Autodesk Inventor part; units mm, degrees
ref_plane "YZ Plane" through (0, 0, 0) normal (1, 0, 0) x (0, 1, 0)
ref_plane "XZ Plane" through (0, 0, 0) normal (0, 1, 0) x (-1, 0, 0)
ref_plane "XY Plane" through (0, 0, 0) normal (0, 0, 1) x (1, 0, 0)
sketch "Sketch1" plane through (0, 0, 0) normal (1, 0, 0) x (0, 1, 0)
  circle A0 centre (0, 0) radius 1.5
  arc A1 (3.5, 0) -> (-3.5, 0) centre (0, 0) ccw
  line L0 (3.5, 0) -> (3.5, -34)
  line L1 (-3.5, 0) -> (-3.5, -34)
  line L2 (-3.5, -34) -> (0, -34)
  circle A2 centre (0, -34) radius 1.5
  arc A3 (-3.5, -34) -> (3.5, -34) centre (0, -34) ccw
  dimension "d0" = 3
  dimension "d1" = 7
  dimension "d2" = 34
  dimension "d3" = 34
  dimension "d4" = 3
extrude "Extrusion1" add sketch "Sketch1" along normal blind 3
properties part number "union_acr"
Source: CAD feature listing. Evaluate the final solid. Frame: model axes, mm. Give positions to 0.01 mm unless a question says otherwise; leave off trailing zeros. Order: outer loops, then holes, each group sorted by start corner. A loop starts at its lowest first (then second) coordinate and runs counter-clockwise, first axis right, second up.
(1) Material intervals for line 1 along Z through (x, y) = (1.65, 0); line 2 along Y through (x, z) = (1.3, -34); line 3 along Z through (x, y) = (1, 1.25), sorted ascending.
(2) Contact query for a flat-ended pin moving along its axis: P1, Ø1.5, axis at x = 1, y = -2, coming from the +Z side. Output: stop coordinate, or through.
(3) Section query A-A (y = 0). Return the cut outline in (x, z), plus the area to 3 significant figures.
(4) Section query D-D (y = 2.25). Return the cut outline in (x, z), plus the area to 3 significant figures.
(5) Section query C-C (z = -33.5). Return the cut outline in (x, y), plus the area to 3 significant figures.
(6) Section query B-B (x = 1.45). Return the cut outline in (y, z), plus the area to 3 significant figures.
(7) Pull-direction query (Y, two-part tool) for faces 1 (the face through (1.48, -1.5, -0.07)), 2 (the face through (1.5, -0.1, 3.5)), 3 (the face through (1, -3.5, -17)); classes: +Y half, -Y half, draft (parallel to the pull), parting line (faces both ways), or undercut.
Outcome:
1. line 1: z = -37.5 to -35.5, -32.5 to -1.5, 1.5 to 3.5
1. line 2: y = -3.5 to -1.5, 1.5 to 3.5
1. line 3: z = -37.27 to -34.83, -33.17 to -0.83, 0.83 to 3.27
2. P1: stops at z = 3.27
3. outline: (0, -37.5) - (3, -37.5) - (3, -35.5) - (0, -35.5) - close; (0, -32.5) - (3, -32.5) - (3, -1.5) - (0, -1.5) - close; (0, 1.5) - (3, 1.5) - (3, 3.5) - (0, 3.5) - close
3. area: 105 mm2
4. outline: (0, -36.68) - (3, -36.68) - (3, 2.68) - (0, 2.68) - close
4. area: 118 mm2
5. outline: (0, -3.5) - (3, -3.5) - (3, -1.41) - (0, -1.41) - close; (0, 1.41) - (3, 1.41) - (3, 3.5) - (0, 3.5) - close
5. area: 12.5 mm2
6. outline: (-3.5, -34) arc R3.5 ccw to (3.5, -34) - (3.5, 0) arc R3.5 ccw to (-3.5, 0) - close; hole circle Ø3 at (0, -34); hole circle Ø3 at (0, 0)
6. area: 262 mm2
7. face 1: undercut
7. face 2: parting line
7. face 3: -Y half
